Build history of the part. All positions in model axes, mm. A direction names the side the tool comes from. Give positions to 0.01 mm unless a question says otherwise; leave off trailing zeros. Order: outer loops, then holes, each group sorted by start corner. A loop starts at its lowest first (then second) coordinate and runs counter-clockwise, first axis right, second up. Notation, with made-up numbers: (0.5, -16.75) - (7.5, -16.75) arc R19 ccw to (7.5, -1.75) - close; hole circle Ø9 at (82.25, 79). An arc over 180 degrees is marked (long way). Write each question's results on one line, items separated by ' | '. Start each with the question number.
from build123d import *

# Parameters (mm, degrees)
BOSS_EXTRU_1_DEPTH      = 9
ESQUISSE2_W             = 15.557161579
ESQUISSE2_H             = 11.468773674
ESQUISSE2_R             = 3
ENL_V_MAT_EXTRU_1_DEPTH = 3
ENL_V_START             = -4
ESQUISSE3_W             = 15.323034965
ESQUISSE3_H             = 11.861185192
ESQUISSE3_R             = 3
ENL_V_MAT_EXTRU_3_DEPTH = 4
CHANFREIN2_SIZE         = 4
CHANFREIN2_SIZE_2       = 2.499477408


with BuildPart() as part:
    # Esquisse1 → Boss.-Extru.1 (new body)
    with BuildSketch(Plane.XY):
        Polygon((4.041451884, 0), (2.020725942, 3.5), (-2.020725942, 3.5), (-4.041451884, 0), (-2.020725942, -3.5), (2.020725942, -3.5), align=None)
    extrude(amount=BOSS_EXTRU_1_DEPTH)

    # Esquisse2 → Enlèv. mat.-Extru.1 (cut)
    with BuildSketch(Plane.XY.offset(9)):
        with Locations((-0.212602531, -0.232116366)):
            Rectangle(ESQUISSE2_W, ESQUISSE2_H)
        Circle(ESQUISSE2_R, mode=Mode.SUBTRACT)
    extrude(amount=-ENL_V_MAT_EXTRU_1_DEPTH, mode=Mode.SUBTRACT)

    # Esquisse3 → Enlèv. mat.-Extru.3 (cut)
    with BuildSketch(Plane(origin=(0, 0, 0), x_dir=(-1, 0, 0), z_dir=(0, 0, -1)).offset(ENL_V_START)):
        with Locations((0.20407301, -0.146192801)):
            Rectangle(ESQUISSE3_W, ESQUISSE3_H)
        with Locations(Location((0, 0, 0), (0, 0, 180))):
            Circle(ESQUISSE3_R, mode=Mode.SUBTRACT)
    extrude(amount=ENL_V_MAT_EXTRU_3_DEPTH, mode=Mode.SUBTRACT)

    # Chanfrein2
    # the kernel refuses this chamfer: 4, 2.499477408 mm, written as the material it takes off along each edge
    with BuildSketch(Plane(origin=(0, 0, 0), x_dir=(1, 0, 0), z_dir=(0, 1, 0))) as chanfrein2_piece_1_section:
        Polygon((3, -CHANFREIN2_SIZE), (3 - CHANFREIN2_SIZE_2, 0), (3, 0), align=None)
    chanfrein2_piece_1 = revolve(axis=Axis((0, 0, 0), (0, 0, -1)), mode=Mode.PRIVATE)
    chanfrein2_piece_1 = split(chanfrein2_piece_1, bisect_by=Plane(origin=(-1.744026904, 0, 4), z_dir=(0, 0, -1)), keep=Keep.TOP, mode=Mode.PRIVATE)
    add(chanfrein2_piece_1, mode=Mode.SUBTRACT)

    # Esquisse4 → Enlèvement de matière-Révolution1 (revolve, cut)
    with BuildSketch(Plane(origin=(0, 0, 0), x_dir=(1, 0, 0), z_dir=(0, 1, 0))):
        Polygon((0, 1.4), (1, -6.6), (1, -9), (0, -9), align=None)
    revolve(axis=Axis((0, 0, 9), (0, 0, -1)), mode=Mode.SUBTRACT)


solid = part.part
Item 1: Cut at B-B, the plane z = 8.5. List the corners of the cut face in (x, y), then the cut area to 3 significant figures.
Item 2: Probe line 1 along Y through (x, z) = (0, 8.55); line 2 along Y through (x, z) = (0.25, 1.75); line 3 along X through (y, z) = (-0.25, 6.5). List the from-to ranges inside material, lowest first. Write a range as from..to.
Item 3: Which spindle directions (+Z, -Z, +X, -X, +Y, -Y) get a long thin tool onto all of the face, cutting with end or side? Do faces 5 (the flat face through (1, 3, 4)), 6 (the flat face through (-1, 1, 9)), 7 (the flat face through (-1, 3, 6)). Say none if no direction does.
Item 4: Flat gauge pin, fed straight in: pin 1 Ø2 at (x, z) = (-2, 1.5) entering from -Y. Where does the tip first touch, or does it go through?
Item 5: Two-plate mould, pull along X, no slides. Class faces 1 (the flat face through (3.045, 1.726, 4.986)), 2 (the flat face through (-3, 1.8, 5)), 3 (the conical face through (0.566, -0.178, 3.346)), 4 (the flat face through (0, -3.5, 5)): +X half, -X half, draft (parallel to the pull), parting line (faces both ways), or undercut.
Item 6: Cut at A-A, the plane x = 0. List the corners of the cut face in (y, z) (3 decimals), then the cut area to 3 significant figures.
Item 7: Cut at C-C, the plane z = 2.5. List the corners of the cut face in (x, y) (1 decimal).
Values found:
1) outline: circle Ø6 at (0, 0); hole circle Ø2 at (0, 0) | area: 25.1 mm2
2) line 1: y = -3..-1, 1..3 | line 2: y = -1.57..-0.3, 0.3..1.57 | line 3: x = -2.99..-0.96, 0.96..2.99
3) face 5: -Z | face 6: +Z, +X, -X, +Y, -Y | face 7: +Z
4) pin 1: stops at y = -1.37
5) face 1: +X half | face 2: -X half | face 3: undercut | face 4: draft
6) outline: (-3.5, 4) - (-3, 4) - (-0.501, 0) - (-0.175, 0) - (-1, 6.6) - (-1, 9) - (-3, 9) - (-3, 6) - (-3.5, 6) - close; (0.175, 0) - (0.501, 0) - (3, 4) - (3.5, 4) - (3.5, 6) - (3, 6) - (3, 9) - (1, 9) - (1, 6.6) - close | area: 33.4 mm2
7) outline: circle Ø4.1 at (0, 0); hole circle Ø1 at (0, 0)
